from build123d import *

# Parameters (mm, degrees)
BOSS_EXTRUDE1_DEPTH = 14.986
SKETCH2_R           = 1.6
CUT_EXTRUDE1_DEPTH  = 25
SKETCH4_R           = 1.6
CUT_EXTRUDE2_DEPTH  = 25


with BuildPart() as part:
    # Sketch1 → Boss-Extrude1 (new body)
    with BuildSketch(Plane(origin=(0, 0, 0), x_dir=(1, 0, 0), z_dir=(0, 1, 0))):
        Polygon((0, 0), (0, 20.32), (20.32, 20.32), (20.32, 17.32), (3, 17.32), (3, 0), align=None)
    extrude(amount=BOSS_EXTRUDE1_DEPTH)

    # Sketch2 → Cut-Extrude1 (cut)
    with BuildSketch(Plane.ZY):
        with Locations((-5.37, 3.55)):
            Circle(SKETCH2_R)
        with Locations((-15.27, 3.55)):
            Circle(SKETCH2_R)
    extrude(amount=-CUT_EXTRUDE1_DEPTH, mode=Mode.SUBTRACT)

    # Sketch4 → Cut-Extrude2 (cut)
    with BuildSketch(Plane.XY.offset(-17.32)):
        with Locations((7.510208413, 7.496)):
            Circle(SKETCH4_R)
        with Locations((15.208779856, 7.493)):
            Circle(SKETCH4_R)
    extrude(amount=-CUT_EXTRUDE2_DEPTH, mode=Mode.SUBTRACT)


solid = part.part
Model file for the job. Use its own axes, mm. A direction names the side the tool comes from. Coordinates: 2 decimals unless noted, no trailing zeros. Write each loop counter-clockwise with the first axis right and the second up, starting at its lowest first coordinate (ties: lowest second). Pieces come first, ordered by that corner, then holes. Notation, with made-up numbers: (82.25, 6.5) -> (120.25, 6.5) arc R25 ccw to (120.25, 45.5) -> close; hole circle Ø1 at (86.5, 67.5). An arc over 180 degrees is marked (long way). One line per item, written item: value. Start each with the question number.
1) Which spindle directions (+Z, -Z, +X, -X, +Y, -Y) get a long thin tool onto all of the face, cutting with end or side? Do faces 1 (the face through (12, 7, -17.32)), 2 (the face through (1.48, 3.62, -6.97)). Say none if no direction does.
2) Slice it at A-A on y = 3.55. Write the cut outline in (x, z).
3) Slice it at D-D on x = 14.75. Write the cut outline in (y, z).
4) Slice it at B-B on z = -15.27. Write the cut outline in (x, y).
5) Probe probe 1 along Y at (x, z) = (2.1, -15.27); probe 2 along Z at (x, y) = (5.75, 1.5); probe 3 along X at (y, z) = (2.5, -1.25). List the from-to ranges inside material, lowest first.
6) Slice it at C-C on x = 1.25. Write the cut outline in (y, z).
7) Pull direction Y, two halves, no side cores. Call faces 3 (the face through (3, 7, -9)), 4 (the face through (6.331, 8.577, -18.799)), 5 (the face through (6, 0, -18)), 6 (the face through (6, 14.986, -18)): +Y half, -Y half, draft (parallel to the pull), parting line (faces both ways), or undercut.
8) Flat gauge pins, fed straight in: pin 1 Ø6 at (x, y) = (9.5, 7.5) entering from +Z; pin 2 Ø4 at (y, z) = (3.55, -15.27) entering from +X. Where does each tip first touch, or does it go through?
Answers follow:
1. face 1: +Z, +X, +Y, -Y
1. face 2: +X, -X
2. outline: (0, -20.32) -> (20.32, -20.32) -> (20.32, -17.32) -> (3, -17.32) -> (3, -16.87) -> (0, -16.87) -> close; (0, -13.67) -> (3, -13.67) -> (3, -6.97) -> (0, -6.97) -> close; (0, -3.77) -> (3, -3.77) -> (3, 0) -> (0, 0) -> close
3. outline: (0, -20.32) -> (5.96, -20.32) -> (5.96, -17.32) -> (0, -17.32) -> close; (9.03, -20.32) -> (14.99, -20.32) -> (14.99, -17.32) -> (9.03, -17.32) -> close
4. outline: (0, 0) -> (3, 0) -> (3, 1.95) -> (0, 1.95) -> close; (0, 5.15) -> (3, 5.15) -> (3, 14.99) -> (0, 14.99) -> close
5. probe 1: 0 to 1.95, 5.15 to 14.99
5. probe 2: -20.32 to -17.32
5. probe 3: 0 to 3
6. outline: (0, -20.32) -> (14.99, -20.32) -> (14.99, 0) -> (0, 0) -> close; hole circle Ø3.2 at (3.55, -15.27); hole circle Ø3.2 at (3.55, -5.37)
7. face 3: draft
7. face 4: undercut
7. face 5: -Y half
7. face 6: +Y half
8. pin 1: z = -17.32
8. pin 2: x = 3
